The model under review builds one solid part; all positions refer to its coordinate system, in mm. Face numbers are marked on the shaded views. A direction names the side the tool comes from. Give positions to 0.01 mm unless a question says otherwise; leave off trailing zeros. Order: outer loops, then holes, each group sorted by start corner. A loop starts at its lowest first (then second) coordinate and runs counter-clockwise, first axis right, second up. Notation, with made-up numbers: (26, 21) -> (48, 21) arc R16 ccw to (48, 51) -> close; hole circle Ø10 at (34.5, 83.25). An arc over 180 degrees is marked (long way). Use one line per item in the form item = value.
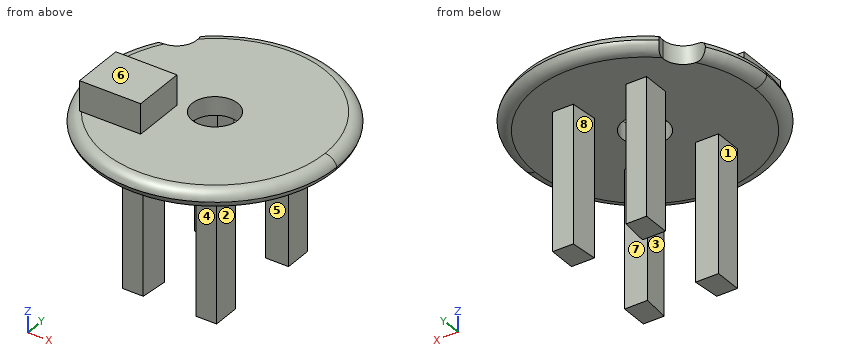
```python
from build123d import *

# Parameters (mm, degrees)
F1_DEPTH    = 7.62
F3_DEPTH    = 57.15
F4_T2_ANGLE = 118.6593978475
F4_T4_ANGLE = 118.6593978475
F7_R        = 8.2517563721
F8_DEPTH    = 25.4
F9_R        = 9.4542856314
F10_DEPTH   = 26.162
F11_W       = 25.4
F11_H       = 21.8551358064
F12_DEPTH   = 12.446


# Not quite as in the source:
# - a fillet or chamfer that OpenCascade refuses, or shapes differently, is made with other operations: its cross-section is extruded or revolved along the edge and cut away or added


with BuildPart() as f1:
    # F0 (on Top) → F1 (new body)
    with BuildSketch(Plane.XY):
        with BuildLine():
            ThreePointArc((0, -50.8), (35.9210244843, -35.9210244843), (50.8, 0))
            Line((50.8, 0), (0, 0))
            Line((0, 0), (0, -50.8))
        make_face()
    extrude(amount=F1_DEPTH)

    # F2 (on face) → F3 (join)
    with BuildSketch(Plane(origin=(0, 0, 0), x_dir=(1, 0, 0), z_dir=(0, 0, -1))):
        Polygon((19.5075478405, 27.366604656), (10.9492652118, 27.366604656), (9.9541153759, 16.0219036043), (19.5075478405, 16.0219036043), align=None)
    extrude(amount=F3_DEPTH)

    # F4: fillet of radius 5.08 on 2 edges, made by hand

    # F4_s1 → F4_t2 (revolve, cut)
    with BuildSketch(Plane(origin=(0, 0, 0), x_dir=(0, 0, 1), z_dir=(-0.9688875708, 0.247501263, 0))):
        with BuildLine():
            ThreePointArc((2.54, -50.8), (6.1321024484, -49.3121024484), (7.62, -45.72))
            Line((7.62, -45.72), (7.62, -50.8))
            Line((7.62, -50.8), (2.54, -50.8))
        make_face()
    revolve(axis=Axis((0, 0, 7.62), (0, 0, 1)), revolution_arc=F4_T2_ANGLE, mode=Mode.SUBTRACT)

    # F4_s3 → F4_t4 (revolve, cut)
    with BuildSketch(Plane(origin=(0, 0, 0), x_dir=(0, 0, 1), z_dir=(-0.9688875708, 0.247501263, 0))):
        with BuildLine():
            ThreePointArc((5.08, -50.8), (1.4878975516, -49.3121024484), (0, -45.72))
            Line((0, -45.72), (0, -50.8))
            Line((0, -50.8), (5.08, -50.8))
        make_face()
    revolve(axis=Axis((0, 0, 0), (0, 0, 1)), revolution_arc=F4_T4_ANGLE, mode=Mode.SUBTRACT)

    # F5: F1 across plane


with BuildPart() as f1_1:
    add(f1.part)
    add(f1.part.mirror(Plane.YZ))

    # F6: F1 across plane


with BuildPart() as f1_2:
    add(f1_1.part)
    add(f1_1.part.mirror(Plane.XZ))

    # F7 (on face) → F8 (cut)
    with BuildSketch(Plane.XY.offset(7.62)):
        with Locations((-38.7037992477, 33.2289077342)):
            Circle(F7_R)
    extrude(amount=-F8_DEPTH, mode=Mode.SUBTRACT)

    # F9 (on face) → F10 (cut)
    with BuildSketch(Plane.XY.offset(7.62)):
        Circle(F9_R)
    extrude(amount=-F10_DEPTH, mode=Mode.SUBTRACT)

    # F11 (on face) → F12 (join)
    with BuildSketch(Plane.XY.offset(7.62)):
        with Locations((-25.7072858512, -14.9798975326)):
            Rectangle(F11_W, F11_H)
    extrude(amount=F12_DEPTH)


solid = f1_2.part
```
1. Add section C-C on z = 13. Give the boundary of the cut face in (x, y), then the cut area to 3 significant figures.
Values:
outline = (-38.41, -25.91) -> (-13.01, -25.91) -> (-13.01, -4.05) -> (-38.41, -4.05) -> close
area = 555 mm^2
2. Add section B-B on z = -13.5. Give the boundary of the cut face in (x, y).
Values:
outline = (-19.51, -27.37) -> (-10.95, -27.37) -> (-9.95, -16.02) -> (-19.51, -16.02) -> close; (-19.51, 16.02) -> (-9.95, 16.02) -> (-10.95, 27.37) -> (-19.51, 27.37) -> close; (9.95, -16.02) -> (10.95, -27.37) -> (19.51, -27.37) -> (19.51, -16.02) -> close; (9.95, 16.02) -> (19.51, 16.02) -> (19.51, 27.37) -> (10.95, 27.37) -> close
3. Tool access review of the marked faces 1, 2, 3, 4 and 5: name each direction out of +Z, -Z, +X, -X, +Y, -Y from which nothing blocks a thin tool from reaching the whole face with its end or side.
Values:
face_1 = -Z, -X, +Y, -Y
face_2 = -Z, +X, +Y, -Y
face_3 = -Z, -Y
face_4 = -Z, +X, -X, -Y
face_5 = -Z, +X, -X
4. The part is to be moulded in two halves that separate along Y. For the marked faces 6, 7 and 8, say which applies: +Y half, -Y half, draft (parallel to the pull), parting line (faces both ways), or undercut.
Values:
face_6 = draft
face_7 = undercut
face_8 = +Y half
5. Add section A-A on x = 0. Give the boundary of the cut face in (y, z), then the cut area to 3 significant figures.
Values:
outline = (-50.64, 3.81) arc R5.08 ccw to (-45.72, 0) -> (-9.45, 0) -> (-9.45, 7.62) -> (-45.72, 7.62) arc R5.08 ccw to start; (9.45, 0) -> (45.72, 0) arc R5.08 ccw to (50.64, 3.81) arc R5.08 ccw to (45.72, 7.62) -> (9.45, 7.62) -> close
area = 608 mm^2
6. For pin 1 Ø3.5 at (x, z) = (-21.5, 11) entering from -Y; pin 2 Ø5 at (x, y) = (-20.5, 4) entering from -Z; pin 3 Ø5 at (x, y) = (-10.5, 23.5) entering from +Z; pin 4 Ø4 at (y, z) = (-13.5, -36.5) entering from -X, all flat-tipped, find the tip position at first contact; note any pin that passes through.
Values:
pin_1 = -25.91
pin_2 = 0
pin_3 = 7.62
pin_4 = through
7. For L1, parallel to Z at x = 26, y = 8.5; L2, parallel to Y at x = -13, z = -18; L3, parallel to X at y = 0, z = 3, list the stretches that pass through material, from the lowest coordinate up.
Values:
L1 = 0 to 7.62
L2 = -27.37 to -16.02, 16.02 to 27.37
L3 = -50.35 to -9.45, 9.45 to 50.35
